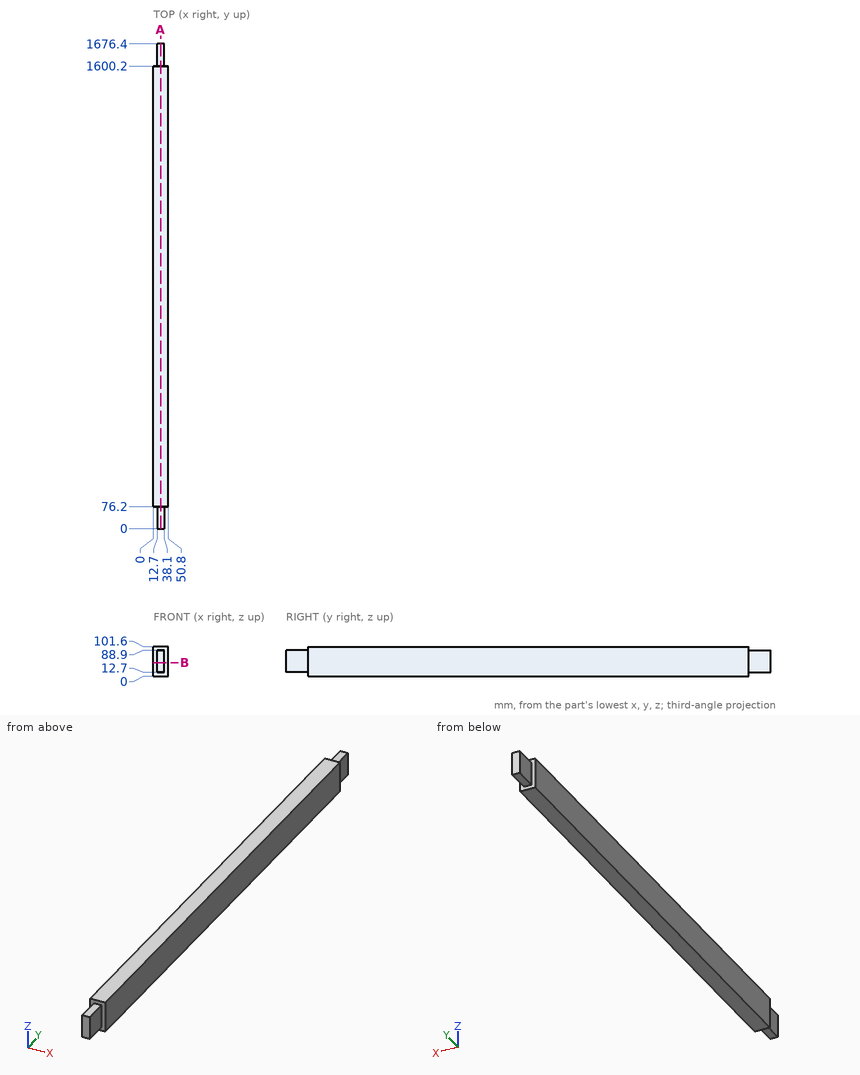
Drawing for the job (mm, zero at the part's lowest x, y, z). Give positions to 0.01 mm unless a question says otherwise; leave off trailing zeros. Order: outer loops, then holes, each group sorted by start corner. A loop starts at its lowest first (then second) coordinate and runs counter-clockwise, first axis right, second up. Notation, with made-up numbers: (54, -32.75) - (73, -32.75) arc R15 cw to (73, -17.75) - close; hole circle Ø4 at (50.5, -19.75). An arc over 180 degrees is marked (long way). Use one line per item in the form item = value.
Item 1: Slice it at A-A on x = 25.5. Give the cut face in (y, z).
Solution:
outline = (0, 12.7) - (76.2, 12.7) - (76.2, 0) - (1600.2, 0) - (1600.2, 12.7) - (1676.4, 12.7) - (1676.4, 88.9) - (1600.2, 88.9) - (1600.2, 101.6) - (76.2, 101.6) - (76.2, 88.9) - (0, 88.9) - close
Item 2: Pin check, flat tips, straight feed: pin 1 Ø8 at (y, z) = (240.5, 59.5) entering from -X; pin 2 Ø20.5 at (x, y) = (30.5, 1633.5) entering from +Z; pin 3 Ø12.5 at (x, y) = (28, 1633.5) entering from -Z. Stop position of each tip, or through.
Solution:
pin_1 = 0
pin_2 = 88.9
pin_3 = 12.7
Item 3: Slice it at B-B on z = 46.5. Give the cut face in (x, y), and give its area (3 significant figures).
Solution:
outline = (0, 76.2) - (12.7, 76.2) - (12.7, 0) - (38.1, 0) - (38.1, 76.2) - (50.8, 76.2) - (50.8, 1600.2) - (38.1, 1600.2) - (38.1, 1676.4) - (12.7, 1676.4) - (12.7, 1600.2) - (0, 1600.2) - close
area = 81,300 mm2
Item 4: Probe probe 1 along Y at (x, z) = (45, 25.5); probe 2 along X at (y, z) = (1608.5, 33). List the from-to ranges inside material, lowest first. Write a range as from..to.
Solution:
probe_1 = 76.2..1600.2
probe_2 = 12.7..38.1
